Model file for the job. Use its own axes, mm. Face numbers are marked on the shaded views. A direction names the side the tool comes from. Give positions to 0.01 mm unless a question says otherwise; leave off trailing zeros. Write each loop counter-clockwise with the first axis right and the second up, starting at its lowest first coordinate (ties: lowest second). Pieces come first, ordered by that corner, then holes.
```python
from build123d import *

# Parameters (mm, degrees)
MAIN_START              = 42
SKETCH1_R               = 32.4
MAIN_JOURNAL_1_DEPTH    = 27.76
MAIN_START_2            = -69.76
SKETCH2_R               = 32.4
MAIN_JOURNAL_2_DEPTH    = 27.76
MAIN_START_3            = -181.52
SKETCH3_R               = 32.4
MAIN_JOURNAL_3_DEPTH    = 27.76
MAIN_START_4            = -293.28
SKETCH4_R               = 32.4
MAIN_JOURNAL_4_DEPTH    = 27.76
MAIN_START_5            = -407
SKETCH5_R               = 32.4
MAIN_JOURNAL_5_DEPTH    = 29.72
SNOUT_START             = 69.76
SKETCH6_R               = 25
SNOUT_DEPTH             = 69.24
FLYWHEEL_START          = -419
SKETCH7_R               = 55
FLYWHEEL_FLANGE_DEPTH   = 12
ROD_START               = -24
SKETCH8_R               = 26.65
ROD_JOURNAL_1_DEPTH     = 48
WEB_START               = 24
WEB_1A_DEPTH            = 18
WEB_START_2             = -42
WEB_1B_DEPTH            = 18
ROD_START_2             = -135.76
SKETCH11_R              = 26.65
ROD_JOURNAL_2_DEPTH     = 48
WEB_START_3             = -87.76
WEB_2A_DEPTH            = 18
WEB_START_4             = -153.76
WEB_2B_DEPTH            = 18
ROD_START_3             = -247.52
SKETCH14_R              = 26.65
ROD_JOURNAL_3_DEPTH     = 48
WEB_START_5             = -199.52
WEB_3A_DEPTH            = 18
WEB_START_6             = -265.52
WEB_3B_DEPTH            = 18
ROD_START_4             = -359.28
SKETCH17_R              = 26.65
ROD_JOURNAL_4_DEPTH     = 48
WEB_START_7             = -311.28
WEB_4A_DEPTH            = 18
WEB_START_8             = -377.28
WEB_4B_DEPTH            = 18
FLANGE_START            = -420
SKETCH20_R              = 5.5
FLANGE_BOLT_HOLES_DEPTH = 13


with BuildPart() as part:
    # Sketch1 → Main Journal 1 (new body)
    with BuildSketch(Plane.XY.offset(MAIN_START)):
        Circle(SKETCH1_R)
    extrude(amount=MAIN_JOURNAL_1_DEPTH)

    # Sketch6 → Snout (add)
    with BuildSketch(Plane.XY.offset(SNOUT_START)):
        Circle(SKETCH6_R)
    extrude(amount=SNOUT_DEPTH)



with BuildPart() as body_2:
    # Sketch2 → Main Journal 2 (new body)
    with BuildSketch(Plane.XY.offset(MAIN_START_2)):
        Circle(SKETCH2_R)
    extrude(amount=MAIN_JOURNAL_2_DEPTH)


with BuildPart() as body_3:
    # Sketch3 → Main Journal 3 (new body)
    with BuildSketch(Plane.XY.offset(MAIN_START_3)):
        with Locations(Location((0, 0, 0), (0, 0, 180))):
            Circle(SKETCH3_R)
    extrude(amount=MAIN_JOURNAL_3_DEPTH)


with BuildPart() as body_4:
    # Sketch4 → Main Journal 4 (new body)
    with BuildSketch(Plane.XY.offset(MAIN_START_4)):
        with Locations(Location((0, 0, 0), (0, 0, 180))):
            Circle(SKETCH4_R)
    extrude(amount=MAIN_JOURNAL_4_DEPTH)


with BuildPart() as body_5:
    # Sketch5 → Main Journal 5 (new body)
    with BuildSketch(Plane.XY.offset(MAIN_START_5)):
        Circle(SKETCH5_R)
    extrude(amount=MAIN_JOURNAL_5_DEPTH)

    # Sketch7 → Flywheel Flange (add)
    with BuildSketch(Plane.XY.offset(FLYWHEEL_START)):
        Circle(SKETCH7_R)
    extrude(amount=FLYWHEEL_FLANGE_DEPTH)


with BuildPart() as body_6:
    # Sketch8 → Rod Journal 1 (new body)
    with BuildSketch(Plane.XY.offset(ROD_START)):
        with Locations((0, 46)):
            Circle(SKETCH8_R)
    extrude(amount=ROD_JOURNAL_1_DEPTH)


with BuildPart() as part_1:
    add(part.part)

    add(body_6.part)  # Web 1A merges body 6
    # Sketch9 → Web 1A (add)
    with BuildSketch(Plane.XY.offset(WEB_START)):
        with BuildLine():
            Line((19.160450761, 74.086956522), (40.575072199, 59.47826087))
            ThreePointArc((40.575072199, 59.47826087), (0, -72), (-40.575072199, 59.47826087))
            Line((-40.575072199, 59.47826087), (-19.160450761, 74.086956522))
            ThreePointArc((-19.160450761, 74.086956522), (0, 80), (19.160450761, 74.086956522))
        make_face()
    extrude(amount=WEB_1A_DEPTH)


    add(body_2.part)  # Web 1B merges body 2
    # Sketch10 → Web 1B (add)
    with BuildSketch(Plane.XY.offset(WEB_START_2)):
        with BuildLine():
            Line((19.160450761, 74.086956522), (40.575072199, 59.47826087))
            ThreePointArc((40.575072199, 59.47826087), (0, -72), (-40.575072199, 59.47826087))
            Line((-40.575072199, 59.47826087), (-19.160450761, 74.086956522))
            ThreePointArc((-19.160450761, 74.086956522), (0, 80), (19.160450761, 74.086956522))
        make_face()
    extrude(amount=WEB_1B_DEPTH)



with BuildPart() as body_5_2:
    # Sketch11 → Rod Journal 2 (new body)
    with BuildSketch(Plane.XY.offset(ROD_START_2)):
        with Locations((46, 0)):
            Circle(SKETCH11_R)
    extrude(amount=ROD_JOURNAL_2_DEPTH)


with BuildPart() as part_2:
    add(part_1.part)

    add(body_5_2.part)  # Web 2A merges body 5 2
    # Sketch12 → Web 2A (add)
    with BuildSketch(Plane.XY.offset(WEB_START_3)):
        with BuildLine():
            Line((74.086956522, -19.160450761), (59.47826087, -40.575072199))
            ThreePointArc((59.47826087, -40.575072199), (-72, 0), (59.47826087, 40.575072199))
            Line((59.47826087, 40.575072199), (74.086956522, 19.160450761))
            ThreePointArc((74.086956522, 19.160450761), (80, 0), (74.086956522, -19.160450761))
        make_face()
    extrude(amount=WEB_2A_DEPTH)


    add(body_3.part)  # Web 2B merges body 3
    # Sketch13 → Web 2B (add)
    with BuildSketch(Plane.XY.offset(WEB_START_4)):
        with BuildLine():
            Line((74.086956522, -19.160450761), (59.47826087, -40.575072199))
            ThreePointArc((59.47826087, -40.575072199), (-72, 0), (59.47826087, 40.575072199))
            Line((59.47826087, 40.575072199), (74.086956522, 19.160450761))
            ThreePointArc((74.086956522, 19.160450761), (80, 0), (74.086956522, -19.160450761))
        make_face()
    extrude(amount=WEB_2B_DEPTH)



with BuildPart() as body_4_2:
    # Sketch14 → Rod Journal 3 (new body)
    with BuildSketch(Plane.XY.offset(ROD_START_3)):
        with Locations((-46, 0)):
            Circle(SKETCH14_R)
    extrude(amount=ROD_JOURNAL_3_DEPTH)


with BuildPart() as part_3:
    add(part_2.part)

    add(body_4_2.part)  # Web 3A merges body 4 2
    # Sketch15 → Web 3A (add)
    with BuildSketch(Plane.XY.offset(WEB_START_5)):
        with BuildLine():
            Line((-74.086956522, 19.160450761), (-59.47826087, 40.575072199))
            ThreePointArc((-59.47826087, 40.575072199), (72, 0), (-59.47826087, -40.575072199))
            Line((-59.47826087, -40.575072199), (-74.086956522, -19.160450761))
            ThreePointArc((-74.086956522, -19.160450761), (-80, 0), (-74.086956522, 19.160450761))
        make_face()
    extrude(amount=WEB_3A_DEPTH)


    add(body_4.part)  # Web 3B merges body 4
    # Sketch16 → Web 3B (add)
    with BuildSketch(Plane.XY.offset(WEB_START_6)):
        with BuildLine():
            Line((-74.086956522, 19.160450761), (-59.47826087, 40.575072199))
            ThreePointArc((-59.47826087, 40.575072199), (72, 0), (-59.47826087, -40.575072199))
            Line((-59.47826087, -40.575072199), (-74.086956522, -19.160450761))
            ThreePointArc((-74.086956522, -19.160450761), (-80, 0), (-74.086956522, 19.160450761))
        make_face()
    extrude(amount=WEB_3B_DEPTH)



with BuildPart() as body_3_2:
    # Sketch17 → Rod Journal 4 (new body)
    with BuildSketch(Plane.XY.offset(ROD_START_4)):
        with Locations((0, -46)):
            Circle(SKETCH17_R)
    extrude(amount=ROD_JOURNAL_4_DEPTH)


with BuildPart() as part_4:
    add(part_3.part)

    add(body_3_2.part)  # Web 4A merges body 3 2
    # Sketch18 → Web 4A (add)
    with BuildSketch(Plane.XY.offset(WEB_START_7)):
        with BuildLine():
            Line((-19.160450761, -74.086956522), (-40.575072199, -59.47826087))
            ThreePointArc((-40.575072199, -59.47826087), (0, 72), (40.575072199, -59.47826087))
            Line((40.575072199, -59.47826087), (19.160450761, -74.086956522))
            ThreePointArc((19.160450761, -74.086956522), (0, -80), (-19.160450761, -74.086956522))
        make_face()
    extrude(amount=WEB_4A_DEPTH)


    add(body_5.part)  # Web 4B merges body 5
    # Sketch19 → Web 4B (add)
    with BuildSketch(Plane.XY.offset(WEB_START_8)):
        with BuildLine():
            Line((-19.160450761, -74.086956522), (-40.575072199, -59.47826087))
            ThreePointArc((-40.575072199, -59.47826087), (0, 72), (40.575072199, -59.47826087))
            Line((40.575072199, -59.47826087), (19.160450761, -74.086956522))
            ThreePointArc((19.160450761, -74.086956522), (0, -80), (-19.160450761, -74.086956522))
        make_face()
    extrude(amount=WEB_4B_DEPTH)

    # Sketch20 → Flange Bolt Holes (cut)
    with BuildSketch(Plane.XY.offset(FLANGE_START)):
        with Locations((42, 0)):
            Circle(SKETCH20_R)
        with Locations((21, 36.373066959)):
            Circle(SKETCH20_R)
        with Locations((-21, 36.373066959)):
            Circle(SKETCH20_R)
        with Locations((-42, 0)):
            Circle(SKETCH20_R)
        with Locations((-21, -36.373066959)):
            Circle(SKETCH20_R)
        with Locations((21, -36.373066959)):
            Circle(SKETCH20_R)
    extrude(amount=FLANGE_BOLT_HOLES_DEPTH, mode=Mode.SUBTRACT)


solid = part_4.part
```
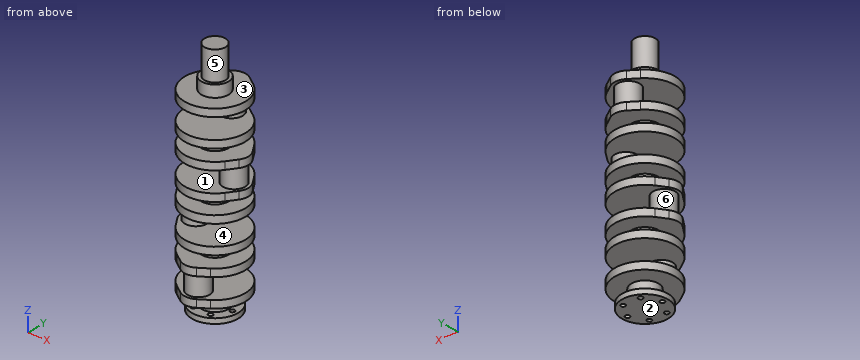
1. Pin check, flat tips, straight feed: P1, Ø12, axis at x = 1.5, z = -87, coming from the +Y side; P2, Ø3, axis at x = 47, y = 36.5, coming from the -Z side; P3, Ø4, axis at x = -14.5, z = -196, coming from the +Y side; P4, Ø17.5, axis at x = -21, y = 36.37, coming from the -Z side. Stop position of each tip, or through.
Calculated:
P1: stops at y = 72
P2: stops at z = -377.28
P3: stops at y = 70.91
P4: stops at z = -419
2. Which spindle directions (+Z, -Z, +X, -X, +Y, -Y) get a long thin tool onto all of the face, cutting with end or side? Do the marked faces 5 and 6. Say none if no direction does.
Calculated:
face 5: +Z
face 6: none
3. Probe probe 1 along Z at (x, y) = (10, 29); probe 2 along Z at (x, y) = (-10, -19); probe 3 along Y at (x, z) = (-21, -414.25). List the from-to ranges inside material, lowest first.
Calculated:
probe 1: z = -419 to -359.28, -311.28 to -247.52, -199.52 to -135.76, -87.76 to 69.76
probe 2: z = -419 to -359.28, -311.28 to -247.52, -199.52 to -135.76, -87.76 to -24, 24 to 139
probe 3: y = -50.83 to -41.87, -30.87 to 30.87, 41.87 to 50.83
4. Slice it at C-C, the plane z = -317. Write the cut outline in (x, y).
Calculated:
outline: circle Ø53.3 at (0, -46)
5. Slice it at A-A, the plane x = 0. State how many separate pieces and enclosed holes the cut face has, and give its area (3 significant figures).
Calculated:
separate pieces: 3
enclosed holes: 0
area: 40,300 mm2
6. Pull direction Z, two halves, no side cores. Call the marked faces 1, 2, 3 and 4: +Z half, -Z half, draft (parallel to the pull), parting line (faces both ways), or undercut.
Calculated:
face 1: undercut
face 2: -Z half
face 3: +Z half
face 4: undercut
7. Slice it at B-B, the plane z = 96.5. Write the cut outline in (x, y), and give its area (3 significant figures).
Calculated:
outline: circle Ø50 at (0, 0)
area: 1,960 mm2
